```python
from build123d import *

# Parameters (mm, degrees)
BASE_FLANGE1_DEPTH             = 2
EDGE_FLANGE1_STRIP_W           = 12
EDGE_FLANGE1_STRIP_H           = 2
EDGE_FLANGE1_STRIP_CUT_DEPTH   = 1422.8
EDGE_FLANGE1_STRIP_2_W         = 12
EDGE_FLANGE1_STRIP_2_H         = 2
EDGE_FLANGE1_STRIP_CUT_2_DEPTH = 110
EDGE_FLANGE1_STRIP_3_W         = 12
EDGE_FLANGE1_STRIP_3_H         = 2
EDGE_FLANGE1_STRIP_CUT_3_DEPTH = 1422.8
EDGE_FLANGE1_STRIP_4_W         = 12
EDGE_FLANGE1_STRIP_4_H         = 2
EDGE_FLANGE1_STRIP_CUT_4_DEPTH = 110
EDGE_FLANGE1_DEPTH             = 1422.8
EDGE_FLANGE1_BEND_DEPTH        = 110
EDGE_FLANGE1_BEND_2_DEPTH      = 1422.8
EDGE_FLANGE1_BEND_3_DEPTH      = 110
FILLET1_R                      = 10


# Sheet-metal steps are written as plain solids
with BuildPart() as part:
    # Sketch1 → Base-Flange1 (new body)
    with BuildSketch(Plane.XY):
        Polygon((-711.4, -100), (711.4, -100), (711.4, -55), (756.4, -55), (756.4, 55), (711.4, 55), (711.4, 100), (-711.4, 100), (-711.4, 55), (-756.4, 55), (-756.4, -55), (-711.4, -55), align=None)
    extrude(amount=-BASE_FLANGE1_DEPTH)

    # Edge-Flange1 strip (across the edge) → Edge-Flange1 strip cut (cut)
    with BuildSketch(Plane(origin=(711.4, 100, 0), x_dir=(0, -1, 0), z_dir=(-1, 0, 0))):
        with Locations((-2, -1)):
            Rectangle(EDGE_FLANGE1_STRIP_W, EDGE_FLANGE1_STRIP_H)
    extrude(amount=EDGE_FLANGE1_STRIP_CUT_DEPTH, mode=Mode.SUBTRACT)

    # Edge-Flange1 strip 2 (across the edge) → Edge-Flange1 strip cut 2 (cut)
    with BuildSketch(Plane(origin=(756.4, -55, 0), x_dir=(-1, 0, 0), z_dir=(0, 1, 0))):
        with Locations((-2, -1)):
            Rectangle(EDGE_FLANGE1_STRIP_2_W, EDGE_FLANGE1_STRIP_2_H)
    extrude(amount=EDGE_FLANGE1_STRIP_CUT_2_DEPTH, mode=Mode.SUBTRACT)

    # Edge-Flange1 strip 3 (across the edge) → Edge-Flange1 strip cut 3 (cut)
    with BuildSketch(Plane(origin=(-711.4, -100, 0), x_dir=(0, 1, 0), z_dir=(1, 0, 0))):
        with Locations((-2, -1)):
            Rectangle(EDGE_FLANGE1_STRIP_3_W, EDGE_FLANGE1_STRIP_3_H)
    extrude(amount=EDGE_FLANGE1_STRIP_CUT_3_DEPTH, mode=Mode.SUBTRACT)

    # Edge-Flange1 strip 4 (across the edge) → Edge-Flange1 strip cut 4 (cut)
    with BuildSketch(Plane(origin=(-756.4, 55, 0), x_dir=(1, 0, 0), z_dir=(0, -1, 0))):
        with Locations((-2, -1)):
            Rectangle(EDGE_FLANGE1_STRIP_4_W, EDGE_FLANGE1_STRIP_4_H)
    extrude(amount=EDGE_FLANGE1_STRIP_CUT_4_DEPTH, mode=Mode.SUBTRACT)

    # Edge-Flange1 section (across the edge) → Edge-Flange1 (add)
    with BuildSketch(Plane(origin=(711.4, 100, 0), x_dir=(0, -1, 0), z_dir=(-1, 0, 0))):
        with BuildLine():
            Line((0, 2), (0, 38))
            Line((0, 38), (2, 38))
            Line((2, 38), (2, 2))
            ThreePointArc((2, 2), (2.585786438, 0.585786438), (4, 0))
            Line((4, 0), (4, -2))
            ThreePointArc((4, -2), (1.171572875, -0.828427125), (0, 2))
        make_face()
    extrude(amount=EDGE_FLANGE1_DEPTH)

    # Edge-Flange1 section 2 (across the edge) → Edge-Flange1 bend (add)
    with BuildSketch(Plane(origin=(756.4, -55, 0), x_dir=(-1, 0, 0), z_dir=(0, 1, 0))):
        with BuildLine():
            Line((0, 2), (0, 38))
            Line((0, 38), (2, 38))
            Line((2, 38), (2, 2))
            ThreePointArc((2, 2), (2.585786438, 0.585786438), (4, 0))
            Line((4, 0), (4, -2))
            ThreePointArc((4, -2), (1.171572875, -0.828427125), (0, 2))
        make_face()
    extrude(amount=EDGE_FLANGE1_BEND_DEPTH)

    # Edge-Flange1 section 3 (across the edge) → Edge-Flange1 bend 2 (add)
    with BuildSketch(Plane(origin=(-711.4, -100, 0), x_dir=(0, 1, 0), z_dir=(1, 0, 0))):
        with BuildLine():
            Line((0, 2), (0, 38))
            Line((0, 38), (2, 38))
            Line((2, 38), (2, 2))
            ThreePointArc((2, 2), (2.585786438, 0.585786438), (4, 0))
            Line((4, 0), (4, -2))
            ThreePointArc((4, -2), (1.171572875, -0.828427125), (0, 2))
        make_face()
    extrude(amount=EDGE_FLANGE1_BEND_2_DEPTH)

    # Edge-Flange1 section 4 (across the edge) → Edge-Flange1 bend 3 (add)
    with BuildSketch(Plane(origin=(-756.4, 55, 0), x_dir=(1, 0, 0), z_dir=(0, -1, 0))):
        with BuildLine():
            Line((0, 2), (0, 38))
            Line((0, 38), (2, 38))
            Line((2, 38), (2, 2))
            ThreePointArc((2, 2), (2.585786438, 0.585786438), (4, 0))
            Line((4, 0), (4, -2))
            ThreePointArc((4, -2), (1.171572875, -0.828427125), (0, 2))
        make_face()
    extrude(amount=EDGE_FLANGE1_BEND_3_DEPTH)

    # Fillet1
    fillet1_edges = [part.edges().sort_by_distance(p)[0] for p in [
        (755.4, -55, 38),
        (755.4, 55, 38),
        (-711.4, -99, 38),
        (711.4, -99, 38),
        (-755.4, 55, 38),
        (-755.4, -55, 38),
        (711.4, 55, -1),
        (711.4, -55, -1),
        (-711.4, -55, -1),
        (-711.4, 55, -1),
        (711.4, 99, 38),
        (-711.4, 99, 38),
    ]]
    fillet(fillet1_edges, radius=FILLET1_R)


solid = part.part
```
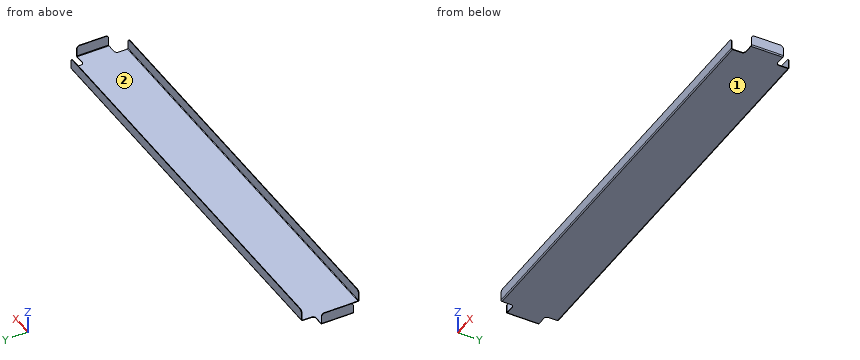
Design review of the part built by this model. Coordinates are the model's own, in mm. Face numbers are marked on the shaded views. Give positions to 0.01 mm unless a question says otherwise; leave off trailing zeros. Write each loop counter-clockwise with the first axis right and the second up, starting at its lowest first coordinate (ties: lowest second). Pieces come first, ordered by that corner, then holes.
(1) Add section A-A (z = 21). Give the boundary of the cut face in (x, y).
Checked values:
outline: (-756.4, -55) - (-754.4, -55) - (-754.4, 55) - (-756.4, 55) - close; (-711.4, -100) - (711.4, -100) - (711.4, -98) - (-711.4, -98) - close; (-711.4, 98) - (711.4, 98) - (711.4, 100) - (-711.4, 100) - close; (754.4, -55) - (756.4, -55) - (756.4, 55) - (754.4, 55) - close
(2) Add section B-B (y = 14). Give the boundary of the cut face in (x, z).
Checked values:
outline: (-756.4, 2) arc R4 ccw to (-752.4, -2) - (752.4, -2) arc R4 ccw to (756.4, 2) - (756.4, 38) - (754.4, 38) - (754.4, 2) arc R2 cw to (752.4, 0) - (-752.4, 0) arc R2 cw to (-754.4, 2) - (-754.4, 38) - (-756.4, 38) - close
(3) Mouldability with a two-part tool opening along X and no side actions: class the marked faces 1 and 2 as +X half, -X half, draft (parallel to the pull), parting line (faces both ways), or undercut.
Checked values:
face 1: draft
face 2: undercut
(4) Wall thickness on line 1 along Y through (x, z) = (-181, 20); line 2 along X through (y, z) = (42.5, 12.5); line 3 along Z through (x, y) = (-197, 87): over which ranges is each line inside the solid? List them lowest first.
Checked values:
line 1: y = -100 to -98, 98 to 100
line 2: x = -756.4 to -754.4, 754.4 to 756.4
line 3: z = -2 to 0
(5) Clearance check with flat-ended pins moving along their axes: pin 1 Ø24 at (y, z) = (-75, 11.5) entering from -X; pin 2 Ø2 at (x, y) = (-97, 42) entering from +Z; pin 3 Ø24 at (y, z) = (-77, 15) entering from +X. State where each tip first meets the part, or that it passes through.
Checked values:
pin 1: stops at x = -711.4
pin 2: stops at z = 0
pin 3: passes through
(6) Add section C-C (x = 102). Give the boundary of the cut face in (y, z), and give its area (3 significant figures).
Checked values:
outline: (-100, 2) arc R4 ccw to (-96, -2) - (96, -2) arc R4 ccw to (100, 2) - (100, 38) - (98, 38) - (98, 2) arc R2 cw to (96, 0) - (-96, 0) arc R2 cw to (-98, 2) - (-98, 38) - (-100, 38) - close
area: 547 mm2
